Geometry check sheet. Reference: the model listing, model coordinates, mm. Face numbers are marked on the shaded views. A direction names the side the tool comes from. Round coordinates to 2 decimals unless told otherwise and drop trailing zeros. Write each loop counter-clockwise with the first axis right and the second up, starting at its lowest first coordinate (ties: lowest second). Pieces come first, ordered by that corner, then holes. Notation, with made-up numbers: M 84,84.5 L 125,84.5 A27 ccw 125,102.5 Z; hole C -22,-28 d9. An arc over 180 degrees is marked long. Use a Markdown table: item, result.
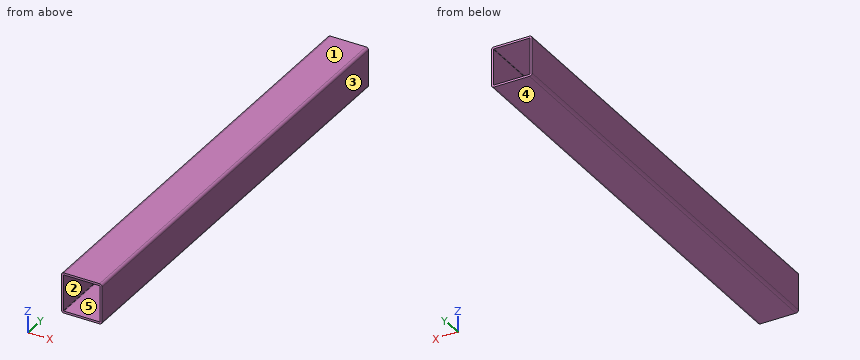
```python
from build123d import *

# Parameters (mm, degrees)
EXTRUDE_1_DEPTH = 900


with BuildPart() as part:
    # Эскиз1 → Вытянуть-Тонкостенный1 (new body)
    with BuildSketch(Plane(origin=(0, 0, 0), x_dir=(1, 0, 0), z_dir=(0, 1, 0))):
        with BuildLine():
            Line((-35, 40), (35, 40))
            ThreePointArc((35, 40), (38.535533906, 38.535533906), (40, 35))
            Line((40, 35), (40, -35))
            ThreePointArc((40, -35), (38.535533906, -38.535533906), (35, -40))
            Line((35, -40), (-35, -40))
            ThreePointArc((-35, -40), (-38.535533906, -38.535533906), (-40, -35))
            Line((-40, -35), (-40, 35))
            ThreePointArc((-40, 35), (-38.535533906, 38.535533906), (-35, 40))
        make_face()
        with BuildLine():
            Line((-35, 36), (35, 36))
            ThreePointArc((35, 36), (35.707106781, 35.707106781), (36, 35))
            Line((36, 35), (36, -35))
            ThreePointArc((36, -35), (35.707106781, -35.707106781), (35, -36))
            Line((35, -36), (-35, -36))
            ThreePointArc((-35, -36), (-35.707106781, -35.707106781), (-36, -35))
            Line((-36, -35), (-36, 35))
            ThreePointArc((-36, 35), (-35.707106781, 35.707106781), (-35, 36))
        make_face(mode=Mode.SUBTRACT)
    extrude(amount=EXTRUDE_1_DEPTH)


solid = part.part
```
Item 1: Access from +Z, -Z, +X, -X, +Y, -Y to the whole of each face (thin tool, end or side, straight path). Record for the marked faces 1 and 2.
Outcome:
| item | result |
|---|---|
| face 1 | +Z, +X, -X, +Y, -Y |
| face 2 | +Y, -Y |
Item 2: Material ranges on line 1 along X through (y, z) = (462, -28), recorded low to high. Write a range as from..to.
Outcome:
| item | result |
|---|---|
| line 1 | x = -40..-36, 36..40 |
Item 3: Cross-section at C-C, the plane y = 703. Record the cut outline in (x, z), and give its area (3 significant figures).
Outcome:
| item | result |
|---|---|
| outline | M -40,-35 A5 ccw -35,-40 L 35,-40 A5 ccw 40,-35 L 40,35 A5 ccw 35,40 L -35,40 A5 ccw -40,35 Z; hole M -36,-35 A1 ccw -35,-36 L 35,-36 A1 ccw 36,-35 L 36,35 A1 ccw 35,36 L -35,36 A1 ccw -36,35 Z |
| area | 1,200 mm2 |
Item 4: Mould release check, pull along Z, two halves, no side actions. Record for the marked faces 3, 4 and 5: +Z half, -Z half, draft (parallel to the pull), parting line (faces both ways), or undercut.
Outcome:
| item | result |
|---|---|
| face 3 | draft |
| face 4 | -Z half |
| face 5 | undercut |
Item 5: Cross-section at B-B, the plane z = -14. Record the cut outline in (x, y), and give its area (3 significant figures).
Outcome:
| item | result |
|---|---|
| outline | M -40,0 L -36,0 L -36,900 L -40,900 Z; M 36,0 L 40,0 L 40,900 L 36,900 Z |
| area | 7,200 mm2 |
Item 6: Cross-section at A-A, the plane x = -27.5. Record the cut outline in (y, z), and give its area (3 significant figures).
Outcome:
| item | result |
|---|---|
| outline | M 0,-40 L 900,-40 L 900,-36 L 0,-36 Z; M 0,36 L 900,36 L 900,40 L 0,40 Z |
| area | 7,200 mm2 |
